Geometry: see drawing. Coordinates: mm, zero at the bounding-box minimum. Give positions to 0.01 mm unless a question says otherwise; leave off trailing zeros. Order: outer loops, then holes, each group sorted by start corner. A loop starts at its lowest first (then second) coordinate and runs counter-clockwise, first axis right, second up. Notation, with made-up numbers: M 81,68 L 122,68 A8 ccw 122,79 Z; hole C 65.5,1.25 d7. An arc over 180 degrees is marked long. Use a Markdown table: item, result.
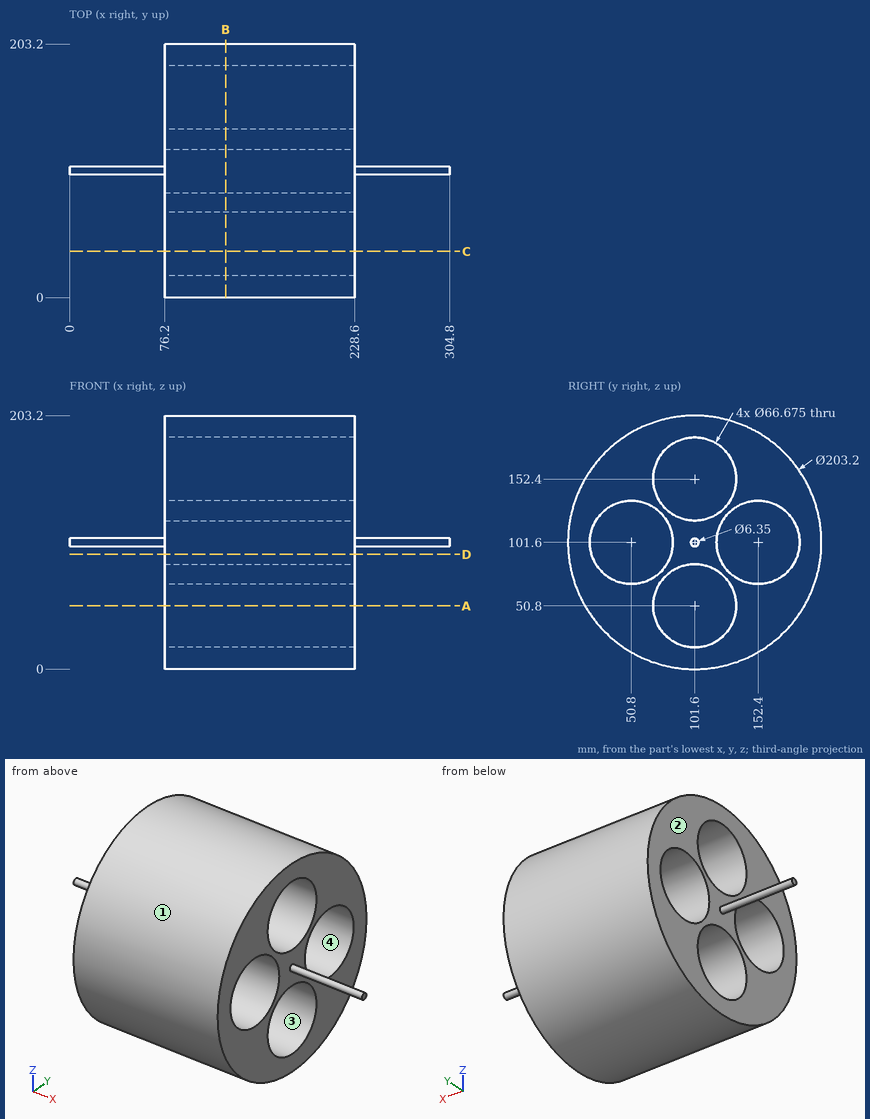
1) Mould query, pull axis Y, two halves, no side actions, for the marked faces 1, 2, 3 and 4. Classes: released by +Y, released by -Y, zero draft, split by the parting line, or undercut.
Response values:
| item | result |
|---|---|
| face 1 | split by the parting line |
| face 2 | zero draft |
| face 3 | undercut |
| face 4 | undercut |
2) Cut plane B-B on x = 125. Return loops of the section in (y, z) (1 decimal), and give its area (3 significant figures).
Response values:
| item | result |
|---|---|
| outline | C 101.6,101.6 d203.2; hole C 50.8,101.6 d66.7; hole C 101.6,50.8 d66.7; hole C 101.6,152.4 d66.7; hole C 152.4,101.6 d66.7 |
| area | 18,500 mm² |
3) Material intervals for line 1 (Z direction, x = 141, y = 102.5); line 2 (Z direction, x = 79, y = 80); line 3 (Z direction, x = 226.5, y = 104.5), sorted ascending. Write a range as from..to.
Response values:
| item | result |
|---|---|
| line 1 | z = 0..17.47, 84.13..119.07, 185.73..203.2 |
| line 2 | z = 2.32..25.41, 76.19..85.51, 117.69..127.01, 177.79..200.88 |
| line 3 | z = 0.04..17.59, 84.01..119.19, 185.61..203.16 |
4) Cut plane C-C on y = 37. Return loops of the section in (x, z), and give its area (3 significant figures).
Response values:
| item | result |
|---|---|
| outline | M 76.2,23.18 L 228.6,23.18 L 228.6,71.25 L 76.2,71.25 Z; M 76.2,131.95 L 228.6,131.95 L 228.6,180.02 L 76.2,180.02 Z |
| area | 14,700 mm² |
5) Cut plane D-D on z = 92. Return loops of the section in (x, y), and give its area (3 significant figures).
Response values:
| item | result |
|---|---|
| outline | M 76.2,0.45 L 228.6,0.45 L 228.6,18.87 L 76.2,18.87 Z; M 76.2,82.73 L 228.6,82.73 L 228.6,120.47 L 76.2,120.47 Z; M 76.2,184.33 L 228.6,184.33 L 228.6,202.75 L 76.2,202.75 Z |
| area | 11,400 mm² |
6) First-contact query: pin 1 Ø6 at (y, z) = (142, 127) entering from +X; pin 2 Ø1.5 at (x, y) = (77, 30.5) entering from +Z; pin 3 Ø6 at (x, y) = (209.5, 152) entering from -Z; pin 4 Ø10 at (x, y) = (232.5, 78.5) entering from +Z. Flat tips, straight axial feed; report the tip coordinate or a pass-through.
Response values:
| item | result |
|---|---|
| pin 1 | passes through |
| pin 2 | stops at z = 174.9 |
| pin 3 | stops at z = 11.73 |
| pin 4 | stops at z = 201.22 |
7) Cut plane A-A on z = 50.8. Return loops of the section in (x, y).
Response values:
| item | result |
|---|---|
| outline | M 76.2,13.61 L 228.6,13.61 L 228.6,68.26 L 76.2,68.26 Z; M 76.2,134.94 L 228.6,134.94 L 228.6,189.59 L 76.2,189.59 Z |
